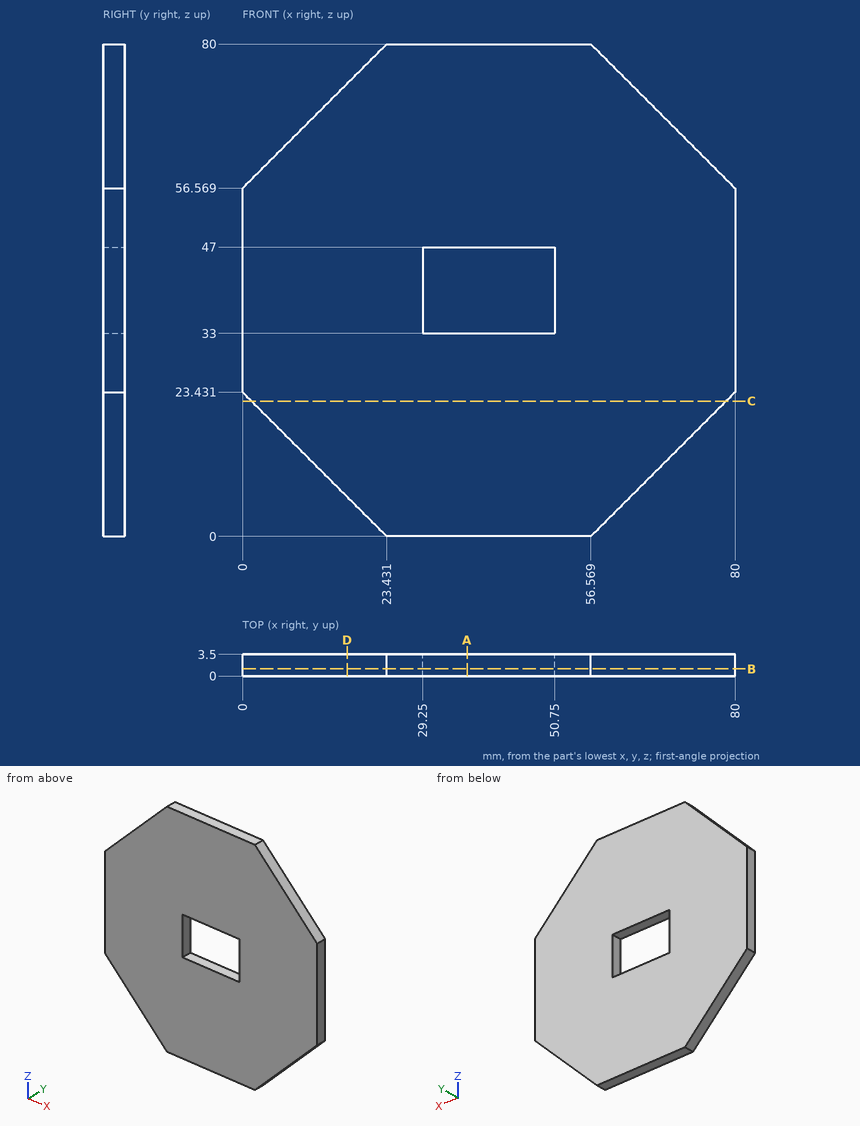
The figure shows three views and two pictorial views of one solid part (mm, origin at its lowest corner). Answer the questions. Round coordinates to 2 decimals unless told otherwise and drop trailing zeros. Write each loop counter-clockwise with the first axis right and the second up, starting at its lowest first coordinate (ties: lowest second). Pieces come first, ordered by that corner, then holes. Notation, with made-up numbers: M 64,67.5 L 82,67.5 A15 ccw 82,87.5 Z; hole C 37.25,-11.75 d7. An arc over 180 degrees is marked long. Use a Markdown table: item, result.
1) Consider line 1 (Z direction, x = 41.5, y = 3.35); line 2 (X direction, y = 0.4, z = 42); line 3 (X direction, y = 2.65, z = 59). Determine where each line is inside the solid, lowest interval first. Write a range as [from, to].
Taken from the geometry:
| item | result |
|---|---|
| line 1 | z = [0, 33], [47, 80] |
| line 2 | x = [0, 29.25], [50.75, 80] |
| line 3 | x = [2.43, 77.57] |
2) The part is cut by section A-A on x = 36.5. Give the vertices of the cut face in (y, z).
Taken from the geometry:
| item | result |
|---|---|
| outline | M 0,0 L 3.5,0 L 3.5,33 L 0,33 Z; M 0,47 L 3.5,47 L 3.5,80 L 0,80 Z |
3) The part is cut by section B-B on y = 1.15. Give the vertices of the cut face in (x, z).
Taken from the geometry:
| item | result |
|---|---|
| outline | M 0,23.43 L 23.43,0 L 56.57,0 L 80,23.43 L 80,56.57 L 56.57,80 L 23.43,80 L 0,56.57 Z; hole M 29.25,33 L 50.75,33 L 50.75,47 L 29.25,47 Z |
4) The part is cut by section D-D on x = 17. Give the vertices of the cut face in (y, z), plus the area to 3 significant figures.
Taken from the geometry:
| item | result |
|---|---|
| outline | M 0,6.43 L 3.5,6.43 L 3.5,73.57 L 0,73.57 Z |
| area | 235 mm2 |
5) The part is cut by section C-C on z = 22. Give the vertices of the cut face in (x, y), plus the area to 3 significant figures.
Taken from the geometry:
| item | result |
|---|---|
| outline | M 1.43,0 L 78.57,0 L 78.57,3.5 L 1.43,3.5 Z |
| area | 270 mm2 |
6) Flat-ended cylindrical pins translate along their axes: pin 1 (1.5 mm diameter, centred on y = 2.5, z = 70, fed in from -X); pin 2 (1 mm diameter, centred on x = 22.5, y = 0.5, fed in from +Z). Find the tip coordinate at first contact, or state that the pin passes through.
Taken from the geometry:
| item | result |
|---|---|
| pin 1 | stops at x = 12.68 |
| pin 2 | stops at z = 79.57 |
